```python
from build123d import *

# Parameters (mm, degrees)
SKIZZE1_R                            = 15
AUFSATZ_LINEAR_AUSTRAGEN1_DEPTH      = 10
AUFSATZ_LINEAR_START                 = -50
SKIZZE4_R                            = 15
AUFSATZ_LINEAR_AUSTRAGEN3_DEPTH      = 50
SCHNITT_LINEAR_AUSTRAGEN1_DEPTH      = 55.313902456
SCHNITT_LINEAR_AUSTRAGEN1_DEPTH_BACK = 55.313902456
SKIZZE5_W                            = 20
SKIZZE5_H                            = 50
SCHNITT_LINEAR_AUSTRAGEN2_DEPTH      = 55.313902456
SCHNITT_LINEAR_AUSTRAGEN2_DEPTH_BACK = 55.313902456
SKIZZE6_R                            = 5


with BuildPart() as part:
    # Skizze1 → Aufsatz-Linear austragen1 (new body)
    with BuildSketch(Plane(origin=(0, 0, 0), x_dir=(1, 0, 0), z_dir=(0, 1, 0))):
        with Locations(Location((0, 0, 0), (0, 0, 270))):
            Circle(SKIZZE1_R)
    extrude(amount=AUFSATZ_LINEAR_AUSTRAGEN1_DEPTH)

    # Skizze4 → Aufsatz-Linear austragen3 (add)
    with BuildSketch(Plane(origin=(0, 0, 0), x_dir=(1, 0, 0), z_dir=(0, 1, 0)).offset(AUFSATZ_LINEAR_START)):
        with Locations(Location((0, 0, 0), (0, 0, 270))):
            Circle(SKIZZE4_R)
    extrude(amount=AUFSATZ_LINEAR_AUSTRAGEN3_DEPTH)

    # Skizze5 → Schnitt-Linear austragen1 (cut, two sides: drawn at the far end of the back side and taken through both)
    with BuildSketch(Plane.XY.offset(-SCHNITT_LINEAR_AUSTRAGEN1_DEPTH_BACK)):
        with Locations((0, -25)):
            Rectangle(SKIZZE5_W, SKIZZE5_H)
    extrude(amount=SCHNITT_LINEAR_AUSTRAGEN1_DEPTH + SCHNITT_LINEAR_AUSTRAGEN1_DEPTH_BACK, mode=Mode.SUBTRACT)

    # Skizze6 → Schnitt-Linear austragen2 (cut, two sides: drawn at the far end of the back side and taken through both)
    with BuildSketch(Plane(origin=(0, 0, 0), x_dir=(0, 0, -1), z_dir=(1, 0, 0)).offset(-SCHNITT_LINEAR_AUSTRAGEN2_DEPTH_BACK)):
        with Locations((0, -40)):
            Circle(SKIZZE6_R)
    extrude(amount=SCHNITT_LINEAR_AUSTRAGEN2_DEPTH + SCHNITT_LINEAR_AUSTRAGEN2_DEPTH_BACK, mode=Mode.SUBTRACT)


solid = part.part
```
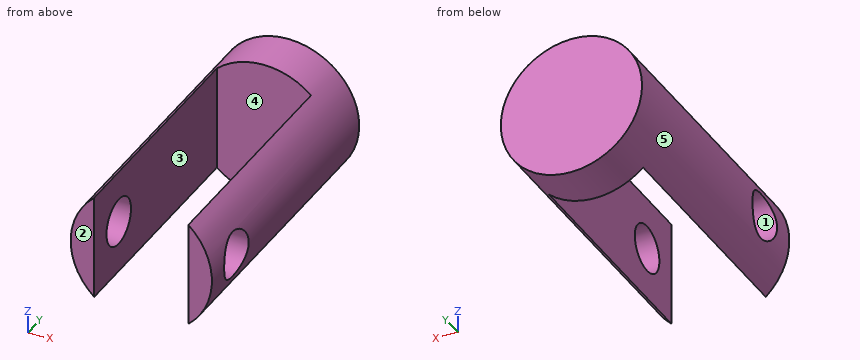
Here's how the part is built. I have some questions about the finished solid (model axes, mm). Face numbers are marked on the shaded views. A direction names the side the tool comes from. Round coordinates to 2 decimals unless told otherwise and drop trailing zeros. Order: outer loops, then holes, each group sorted by start corner. A loop starts at its lowest first (then second) coordinate and runs counter-clockwise, first axis right, second up. Notation, with made-up numbers: M 7,62 L 29,62 A23 cw 29,98 Z; hole C 10.25,-28.75 d5. An arc over 180 degrees is marked long. Answer as CSV lines item,"result".
Item 1: Please list where these lines run through material, in increasing order: L1, parallel to Y at x = 13.3, z = 0; L2, parallel to X at y = -23.5, z = 0.5; L3, parallel to Y at x = -6, z = -0.5. Write a range as [from, to].
From the geometry:
L1,"[-50, -45], [-35, 10]"
L2,"[-14.99, -10], [10, 14.99]"
L3,"[0, 10]"
Item 2: We'd pull the mould along Y, two halves only. Please class the marked faces 1, 2 and 3: +Y half, -Y half, draft (parallel to the pull), parting line (faces both ways), or undercut.
From the geometry:
face 1,"undercut"
face 2,"-Y half"
face 3,"draft"
Item 3: Imagine slicing it at A-A on z = 0. List the corners of the cut face in (x, y) for me.
From the geometry:
outline,"M -15,-50 L -10,-50 L -10,-45 L -15,-45 Z; M -15,-35 L -10,-35 L -10,0 L 10,0 L 10,-35 L 15,-35 L 15,10 L -15,10 Z; M 10,-50 L 15,-50 L 15,-45 L 10,-45 Z"
Item 4: Imagine slicing it at B-B on y = -40. List the corners of the cut face in (x, z) for me, and give its area (3 significant figures).
From the geometry:
outline,"M -14.14,-5 A15 ccw -10,-11.18 L -10,-5 Z; M -14.14,5 L -10,5 L -10,11.18 A15 ccw Z; M 10,-11.18 A15 ccw 14.14,-5 L 10,-5 Z; M 10,5 L 14.14,5 A15 ccw 10,11.18 Z"
area,"60.5 mm2"
Item 5: For pin 1 (1 mm diameter, centred on x = 3, z = -3, fed in from -Y); pin 2 (9 mm diameter, centred on y = -40, z = 0, fed in from +X); pin 3 (8 mm diameter, centred on y = -0.5, z = -5, fed in from -X); pin 4 (3 mm diameter, centred on y = -16.5, z = 10, fed in from +X), each with a flat end and sliding along its axis, tell me the tip position at first contact or that it passes through.
From the geometry:
pin 1,"y = 0"
pin 2,"through"
pin 3,"x = -14.97"
pin 4,"x = 12.36"
Item 6: Imagine slicing it at D-D on x = 0. List the corners of the cut face in (y, z) for me, and give its area (3 significant figures).
From the geometry:
outline,"M 0,-15 L 10,-15 L 10,15 L 0,15 Z"
area,"300 mm2"
Item 7: Imagine slicing it at C-C on y = -18.5. List the corners of the cut face in (x, z) for me.
From the geometry:
outline,"M -10,-11.18 L -10,11.18 A15 ccw Z; M 10,-11.18 A15 ccw 10,11.18 Z"
Item 8: Which directions (+Z, -Z, +X, -X, +Y, -Y) give clear straight access to the entire face, cutting with the end or side of a thin tool? Please do the marked faces 4 and 5.
From the geometry:
face 4,"+Z, -Z, -Y"
face 5,"+Y, -Y"
